from build123d import *

# Parameters (mm, degrees)
SKETCH1_R           = 27.5
SKETCH1_R_2         = 2.0193
BOSS_EXTRUDE1_DEPTH = 2.5
SKETCH2_R           = 17.46
BOSS_EXTRUDE2_DEPTH = 2
CHAMFER5_SIZE       = 1
SKETCH6_R           = 15
BOSS_EXTRUDE3_DEPTH = 30


with BuildPart() as part:
    # Sketch1 → Boss-Extrude1 (new body)
    with BuildSketch(Plane(origin=(0, 0, 0), x_dir=(0, 0, -1), z_dir=(1, 0, 0))):
        Circle(SKETCH1_R)
        with Locations((0, 20.64)):
            Circle(SKETCH1_R_2, mode=Mode.SUBTRACT)
        with Locations((17.874764334, 10.32)):
            Circle(SKETCH1_R_2, mode=Mode.SUBTRACT)
        with Locations((17.874764334, -10.32)):
            Circle(SKETCH1_R_2, mode=Mode.SUBTRACT)
        with Locations((0, -20.64)):
            Circle(SKETCH1_R_2, mode=Mode.SUBTRACT)
        with Locations((-17.874764334, -10.32)):
            Circle(SKETCH1_R_2, mode=Mode.SUBTRACT)
        with Locations((-17.874764334, 10.32)):
            Circle(SKETCH1_R_2, mode=Mode.SUBTRACT)
    extrude(amount=BOSS_EXTRUDE1_DEPTH)

    # Sketch2 → Boss-Extrude2 (add)
    with BuildSketch(Plane.ZY):
        with Locations(Location((0, 0, 0), (0, 0, 180))):
            Circle(SKETCH2_R)
    extrude(amount=BOSS_EXTRUDE2_DEPTH)

    # Chamfer5
    chamfer5_edges = [part.edges().sort_by_distance(p)[0] for p in [
        (-2, 0, 17.46),
    ]]
    chamfer(chamfer5_edges, length=CHAMFER5_SIZE)

    # Sketch6 → Boss-Extrude3 (add)
    with BuildSketch(Plane(origin=(-2, 0, 0), x_dir=(0, 0, -1), z_dir=(1, 0, 0))):
        Circle(SKETCH6_R)
    extrude(amount=-BOSS_EXTRUDE3_DEPTH)


solid = part.part
Design review of the part built by this model. Coordinates are the model's own, in mm. A direction names the side the tool comes from. Round coordinates to 2 decimals unless told otherwise and drop trailing zeros. Write each loop counter-clockwise with the first axis right and the second up, starting at its lowest first coordinate (ties: lowest second). Pieces come first, ordered by that corner, then holes. Notation, with made-up numbers: M 29.25,25.25 L 70.25,25.25 A32 cw 70.25,60.25 Z; hole C -2.75,-20 d11. An arc over 180 degrees is marked long. One line per item, written item: value. Start each with the question number.
1. Take a section at A-A on z = 0. State the section outline as (x, y) points.
2. Take a section at D-D on x = -23. State the section outline as (y, z) points.
3. Take a section at B-B on y = 0. State the section outline as (x, z) points, then the cut area to 3 significant figures.
4. Draft analysis for pull direction Y (two halves, no side actions). For faces 1 (the face through (1.232, -8.955, 19.363)), 2 (the face through (1.232, -26.846, 5.961)), 3 (the face through (2.5, 0, 0)), 4 (the face through (1.23, 18.67, 0.44)), state which applies: pulls with the +Y half, pulls with the -Y half, needs draft (parallel to the pull), parting line crosses it, or undercut.
5. Clearance check with flat-ended pins moving along their axes: P1, Ø10, axis at x = -23.5, z = -18.5, coming from the -Y side; P2, Ø2.5, axis at y = -20.64, z = 0, coming from the +X side; P3, Ø4.5, axis at y = -10.32, z = -17.87, coming from the -X side; P4, Ø1, axis at y = 12, z = 10, coming from the -X side. State where each tip first meets the part, or that it passes through.
6. For faces 5 (the face through (1.232, 10.409, -15.857)), 6 (the face through (-16.79, 0.66, 14.985)), list the 3-axis set-ups (+Z, -Z, +X, -X, +Y, -Y) from which the entire face can be reached by the end or side of a thin tool; tool diameter is ignored.
7. Take a section at C-C on y = 20.64. State the section outline as (x, z) points, then the cut area to 3 significant figures.
8. To check wall thickness, follow probe 1 along Y at (x, z) = (0.65, 0); probe 2 along Z at (x, y) = (1, -10); probe 3 along X at (y, z) = (20.5, -8). State the ranges of each line that lie inside material, in increasing order. Write a range as from..to.
Computed:
1. outline: M -32,-15 L -2,-15 L -2,-16.46 L -1,-17.46 L 0,-17.46 L 0,-18.62 L 2.5,-18.62 L 2.5,18.62 L 0,18.62 L 0,17.46 L -1,17.46 L -2,16.46 L -2,15 L -32,15 Z; M 0,-27.5 L 2.5,-27.5 L 2.5,-22.66 L 0,-22.66 Z; M 0,22.66 L 2.5,22.66 L 2.5,27.5 L 0,27.5 Z
2. outline: C 0,0 d30
3. outline: M -32,-15 L -2,-15 L -2,-16.46 L -1,-17.46 L 0,-17.46 L 0,-27.5 L 2.5,-27.5 L 2.5,27.5 L 0,27.5 L 0,17.46 L -1,17.46 L -2,16.46 L -2,15 L -32,15 Z
3. area: 1,110 mm²
4. face 1: undercut
4. face 2: parting line crosses it
4. face 3: needs draft
4. face 4: undercut
5. P1: stops at y = -6.54
5. P2: passes through
5. P3: stops at x = 0
5. P4: stops at x = -2
6. face 5: +X, -X
6. face 6: -X
7. outline: M 0,-18.17 L 2.5,-18.17 L 2.5,-2.02 L 0,-2.02 Z; M 0,2.02 L 2.5,2.02 L 2.5,18.17 L 0,18.17 Z
7. area: 80.8 mm²
8. probe 1: y = -27.5..-22.66, -18.62..18.62, 22.66..27.5
8. probe 2: z = -25.62..-19.87, -15.88..15.88, 19.87..25.62
8. probe 3: x = 0..2.5
